Part model, mm, in its own coordinate system. A direction names the side the tool comes from. Round coordinates to 2 decimals unless told otherwise and drop trailing zeros. Loops run counter-clockwise (first coordinate to the right, second up) from the corner with the lowest first, then second, coordinate; pieces in that order, holes last.
from build123d import *

# Parameters (mm, degrees)
SKETCH1_W           = 10
SKETCH1_H           = 5
SKETCH1_W_2         = 8
SKETCH1_H_2         = 3
BOSS_EXTRUDE1_DEPTH = 6
BOSS_EXTRUDE2_REACH = 11
SKETCH2_W           = 3
SKETCH2_H           = 1
SKETCH4_R           = 1.5
SKETCH4_R_2         = 1
BOSS_EXTRUDE3_DEPTH = 1
BOSS_EXTRUDE4_DEPTH = 5
BOSS_EXTRUDE5_DEPTH = 5
CUT_EXTRUDE2_DEPTH  = 5
CUT_EXTRUDE3_DEPTH  = 0.333333333
SKETCH8_R           = 2
CUT_EXTRUDE4_DEPTH  = 0.333333333


with BuildPart() as part:
    # Sketch1 → Boss-Extrude1 (new body)
    with BuildSketch(Plane(origin=(0, 0, 0), x_dir=(1, 0, 0), z_dir=(0, 1, 0))):
        with Locations((5, 2.5)):
            Rectangle(SKETCH1_W, SKETCH1_H)
        with Locations((5, 2.5)):
            Rectangle(SKETCH1_W_2, SKETCH1_H_2, mode=Mode.SUBTRACT)
    extrude(amount=BOSS_EXTRUDE1_DEPTH)

    # Sketch2 → Boss-Extrude2 (add, up to next)
    with BuildSketch(Plane(origin=(1, 0, 0), x_dir=(0, 0, -1), z_dir=(1, 0, 0)), mode=Mode.PRIVATE) as boss_extrude2_sk1:
        with Locations((2.5, 5.5)):
            Rectangle(SKETCH2_W, SKETCH2_H)
    boss_extrude2_tool1 = extrude(boss_extrude2_sk1.sketch, amount=BOSS_EXTRUDE2_REACH, mode=Mode.PRIVATE) - part.part
    add(boss_extrude2_tool1.solids().sort_by_distance((1, 5.5, -2.5))[0])

    # Sketch4 → Boss-Extrude3 (add)
    with BuildSketch(Plane(origin=(0, 6, 0), x_dir=(1, 0, 0), z_dir=(0, 1, 0))):
        with Locations((2.5, 2.5)):
            Circle(SKETCH4_R)
        with Locations((2.5, 2.5)):
            Circle(SKETCH4_R_2, mode=Mode.SUBTRACT)
        with Locations((7.5, 2.5)):
            Circle(SKETCH4_R)
        with Locations((7.5, 2.5)):
            Circle(SKETCH4_R_2, mode=Mode.SUBTRACT)
    extrude(amount=BOSS_EXTRUDE3_DEPTH)

    # Sketch6 → Boss-Extrude4 (add)
    with BuildSketch(Plane(origin=(0, 5, 0), x_dir=(-1, 0, 0), z_dir=(0, -1, 0))):
        with BuildLine():
            ThreePointArc((-6, 2.5), (-5, 1.5), (-4, 2.5))
            Line((-4, 2.5), (-6, 2.5))
        make_face()
        with BuildLine():
            Line((-6, 2.5), (-4, 2.5))
            ThreePointArc((-4, 2.5), (-5, 3.5), (-6, 2.5))
        make_face()
    extrude(amount=BOSS_EXTRUDE4_DEPTH)

    # Sketch7 → Boss-Extrude5 (add)
    with BuildSketch(Plane(origin=(0, 0, -5), x_dir=(-1, 0, 0), z_dir=(0, 0, -1))):
        with BuildLine():
            ThreePointArc((-5, 5.5), (-7, 3.5), (-5, 1.5))
            Line((-5, 1.5), (-5, 2))
            ThreePointArc((-5, 2), (-6.5, 3.5), (-5, 5))
            Line((-5, 5), (-5, 5.5))
        make_face()
        with BuildLine():
            Line((-5, 2), (-5, 1.5))
            ThreePointArc((-5, 1.5), (-3.585786438, 2.085786438), (-3, 3.5))
            ThreePointArc((-3, 3.5), (-3.585786438, 4.914213562), (-5, 5.5))
            Line((-5, 5.5), (-5, 5))
            ThreePointArc((-5, 5), (-3.939339828, 4.560660172), (-3.5, 3.5))
            ThreePointArc((-3.5, 3.5), (-3.939339828, 2.439339828), (-5, 2))
        make_face()
        with BuildLine():
            ThreePointArc((-5, 5), (-6.5, 3.5), (-5, 2))
            Line((-5, 2), (-5, 5))
        make_face()
        with BuildLine():
            Line((-5, 5), (-5, 2))
            ThreePointArc((-5, 2), (-3.939339828, 2.439339828), (-3.5, 3.5))
            ThreePointArc((-3.5, 3.5), (-3.939339828, 4.560660172), (-5, 5))
        make_face()
    extrude(amount=-BOSS_EXTRUDE5_DEPTH)

    # Sketch7<3> → Cut-Extrude2 (cut)
    with BuildSketch(Plane(origin=(0, 0, -5), x_dir=(-1, 0, 0), z_dir=(0, 0, -1))):
        with BuildLine():
            ThreePointArc((-5, 5), (-6.5, 3.5), (-5, 2))
            Line((-5, 2), (-5, 5))
        make_face()
        with BuildLine():
            Line((-5, 5), (-5, 2))
            ThreePointArc((-5, 2), (-3.939339828, 2.439339828), (-3.5, 3.5))
            ThreePointArc((-3.5, 3.5), (-3.939339828, 4.560660172), (-5, 5))
        make_face()
    extrude(amount=-CUT_EXTRUDE2_DEPTH, mode=Mode.SUBTRACT)

    # Sketch7<4> → Cut-Extrude3 (cut)
    with BuildSketch(Plane(origin=(0, 0, -5), x_dir=(-1, 0, 0), z_dir=(0, 0, -1))):
        with BuildLine():
            ThreePointArc((-5, 5.5), (-7, 3.5), (-5, 1.5))
            Line((-5, 1.5), (-5, 2))
            ThreePointArc((-5, 2), (-6.5, 3.5), (-5, 5))
            Line((-5, 5), (-5, 5.5))
        make_face()
        with BuildLine():
            Line((-5, 2), (-5, 1.5))
            ThreePointArc((-5, 1.5), (-3.585786438, 2.085786438), (-3, 3.5))
            ThreePointArc((-3, 3.5), (-3.585786438, 4.914213562), (-5, 5.5))
            Line((-5, 5.5), (-5, 5))
            ThreePointArc((-5, 5), (-3.939339828, 4.560660172), (-3.5, 3.5))
            ThreePointArc((-3.5, 3.5), (-3.939339828, 2.439339828), (-5, 2))
        make_face()
    extrude(amount=-CUT_EXTRUDE3_DEPTH, mode=Mode.SUBTRACT)

    # Sketch8 → Cut-Extrude4 (cut)
    with BuildSketch(Plane.XY):
        with Locations((5, 3.5)):
            Circle(SKETCH8_R)
    extrude(amount=-CUT_EXTRUDE4_DEPTH, mode=Mode.SUBTRACT)


solid = part.part
1) Wall check: line 1 along X through (y, z) = (6.4, -2.5); line 2 along X through (y, z) = (3.5, -3.85); line 3 along Z through (x, y) = (2.5, 6.8). Give the ranges that are in metal, low to high.
Values:
line 1: x = 1 to 1.5, 3.5 to 4, 6 to 6.5, 8.5 to 9
line 2: x = 0 to 1, 3 to 3.5, 6.5 to 7, 9 to 10
line 3: z = -4 to -3.5, -1.5 to -1
2) Tool access for faces 1 (the face through (4, 5, -4.667)), 2 (the face through (6, 5, -0.333)), 3 (the face through (6.5, 6.5, -2.5)), 4 (the face through (4.046, 0.896, -2.8)), 5 (the face through (8, 5, -2)): list every direction of +Z, -Z, +X, -X, +Y, -Y with a clear straight run to the whole face (end or side of a thin tool).
Values:
face 1: -Z
face 2: +Z
face 3: +Y
face 4: -Y
face 5: none
3) Mould opens along Z. For faces 6 (the face through (4.9, 0, -4.2)), 7 (the face through (3.8, 1.6, -5)), 8 (the face through (2.175, 6.493, -1.036)), 9 (the face through (2, 6, -2)) say: released by +Z, released by -Z, zero draft, split by the parting line, or undercut.
Values:
face 6: zero draft
face 7: released by -Z
face 8: split by the parting line
face 9: undercut
4) Slice it at C-C, the plane x = 2.5. Give the cut face in (y, z), then the cut area to 3 significant figures.
Values:
outline: (0, -5) - (6, -5) - (6, -4) - (7, -4) - (7, -3.5) - (6, -3.5) - (6, -1.5) - (7, -1.5) - (7, -1) - (6, -1) - (6, 0) - (0, 0) - (0, -1) - (5, -1) - (5, -4) - (0, -4) - close
area: 16.0 mm2
5) Drop flat-ended pins along their axis: pin 1 Ø1.5 at (x, y) = (5.5, 3.5) entering from +Z; pin 2 Ø1 at (x, z) = (2.5, -2.5) entering from +Y. Give the stop position or say it passes through.
Values:
pin 1: passes through
pin 2: stops at y = 6
6) Slice it at D-D, the plane x = 4.75. Give the cut face in (y, z).
Values:
outline: (0, -5) - (1.52, -5) - (1.52, -4.67) - (2.02, -4.67) - (2.02, -0.33) - (1.52, -0.33) - (1.52, 0) - (0, 0) - (0, -1) - (1.52, -1) - (1.52, -1.53) - (0, -1.53) - (0, -3.47) - (1.52, -3.47) - (1.52, -4) - (0, -4) - close; (4.98, -4.67) - (5.48, -4.67) - (5.48, -5) - (6, -5) - (6, 0) - (5.48, 0) - (5.48, -0.33) - (4.98, -0.33) - close
7) Slice it at A-A, the plane y = 4.75. Give the cut face in (x, z).
Values:
outline: (0, -5) - (3.44, -5) - (3.44, -4.67) - (4.17, -4.67) - (4.17, -0.33) - (3.44, -0.33) - (3.44, 0) - (0, 0) - close; (5.83, -4.67) - (6.56, -4.67) - (6.56, -5) - (10, -5) - (10, 0) - (6.56, 0) - (6.56, -0.33) - (5.83, -0.33) - close; hole (1, -4) - (3.44, -4) - (3.44, -1) - (1, -1) - close; hole (6.56, -4) - (9, -4) - (9, -1) - (6.56, -1) - close
